from build123d import *

# Parameters (mm, degrees)
SKETCH1_W             = 74.422
SKETCH1_H             = 50.8
BOSS_EXTRUDE1_DEPTH   = 6.35
SKETCH2_R             = 3.175
CUT_EXTRUDE1_DEPTH    = 64.289975675
SKETCH3_R             = 4.7625
CUT_EXTRUDE2_DEPTH    = 64.289975675
F_8_CLEARANCE_HOLE1_D = 4.4958
SKETCH6_R             = 3.429
CUT_EXTRUDE3_DEPTH    = 4.572
SKETCH7_R             = 1.5875
CUT_EXTRUDE4_DEPTH    = 46.498802413
BODY_MOVE_COPY3_ANGLE = 180


with BuildPart() as part:
    # Sketch1 → Boss-Extrude1 (new body)
    with BuildSketch(Plane(origin=(0, 0, 0), x_dir=(1, 0, 0), z_dir=(0, 1, 0))):
        Rectangle(SKETCH1_W, SKETCH1_H)
    extrude(amount=BOSS_EXTRUDE1_DEPTH)

    # Sketch2 → Cut-Extrude1 (cut, through all)
    with BuildSketch(Plane.XY.offset(25.4)):
        with Locations((-24.511, 0)):
            Circle(SKETCH2_R)
        with Locations((26.289, 0)):
            Circle(SKETCH2_R)
    extrude(amount=-CUT_EXTRUDE1_DEPTH, mode=Mode.SUBTRACT)

    # Sketch3 → Cut-Extrude2 (cut, through all)
    with BuildSketch(Plane.XY.offset(25.4)):
        with Locations((-9.525, 0)):
            Circle(SKETCH3_R)
        with Locations((9.525, 0)):
            Circle(SKETCH3_R)
    extrude(amount=-CUT_EXTRUDE2_DEPTH, mode=Mode.SUBTRACT)

    # #8 Clearance Hole1 (through all)
    with Locations(Plane(origin=(0, 6.35, 0), x_dir=(1, 0, 0), z_dir=(0, 1, 0))):
        with Locations((-32.4485, 12.7), (-32.4485, -12.7), (-17.399, -12.7), (0, -12.7), (17.399, -12.7), (32.4485, -12.7), (32.4485, 12.7), (17.399, 12.7), (0, 12.7), (-17.399, 12.7)):
            Hole(F_8_CLEARANCE_HOLE1_D / 2)

    # Sketch6 → Cut-Extrude3 (cut)
    with BuildSketch(Plane(origin=(0, 6.35, 0), x_dir=(1, 0, 0), z_dir=(0, 1, 0))):
        with Locations(Location((-32.4485, 12.7, 0), (0, 0, 270))):
            Circle(SKETCH6_R)
        with Locations(Location((-17.399, 12.7, 0), (0, 0, 270))):
            Circle(SKETCH6_R)
        with Locations(Location((0, 12.7, 0), (0, 0, 270))):
            Circle(SKETCH6_R)
        with Locations(Location((17.399, 12.7, 0), (0, 0, 270))):
            Circle(SKETCH6_R)
        with Locations(Location((32.4485, 12.7, 0), (0, 0, 270))):
            Circle(SKETCH6_R)
        with Locations(Location((32.4485, -12.7, 0), (0, 0, 270))):
            Circle(SKETCH6_R)
        with Locations(Location((17.399, -12.7, 0), (0, 0, 270))):
            Circle(SKETCH6_R)
        with Locations(Location((0, -12.7, 0), (0, 0, 270))):
            Circle(SKETCH6_R)
        with Locations(Location((-17.399, -12.7, 0), (0, 0, 270))):
            Circle(SKETCH6_R)
        with Locations(Location((-32.4485, -12.7, 0), (0, 0, 270))):
            Circle(SKETCH6_R)
    extrude(amount=-CUT_EXTRUDE3_DEPTH, mode=Mode.SUBTRACT)

    # Sketch7 → Cut-Extrude4 (cut, through all)
    with BuildSketch(Plane(origin=(0, 6.35, 0), x_dir=(1, 0, 0), z_dir=(0, 1, 0))):
        with Locations(Location((0, 0, 0), (0, 0, 270))):
            Circle(SKETCH7_R)
    extrude(amount=-CUT_EXTRUDE4_DEPTH, mode=Mode.SUBTRACT)


with BuildPart() as part_1:
    # Body-Move/Copy3: moved
    add(part.part.moved(Location((0, 0, 0))).rotate(Axis((0, 3.175, 0), (0.7071067811865488, 0, -0.7071067811865462)), BODY_MOVE_COPY3_ANGLE))


solid = part_1.part
Geometry check sheet. Reference: the model listing, model coordinates, mm. A direction names the side the tool comes from. Give positions to 0.01 mm unless a question says otherwise; leave off trailing zeros. Order: outer loops, then holes, each group sorted by start corner. A loop starts at its lowest first (then second) coordinate and runs counter-clockwise, first axis right, second up.
1) Material ranges on probe 1 along X at (y, z) = (1.5, -17.5); probe 2 along X at (y, z) = (3.75, -0.5); probe 3 along Z at (x, y) = (-21, 4.75), recorded low to high.
Results are:
probe 1: x = -25.4 to -16.13, -9.27 to 9.27, 16.13 to 25.4
probe 2: x = -25.4 to -16.09, -9.31 to -1.51, 1.51 to 9.31, 16.09 to 25.4
probe 3: z = -37.21 to -29.03, -23.55 to -14.01, -5.04 to 5.04, 14.01 to 21.77, 27.25 to 37.21
2) Cross-section at A-A (z = 0). Record the boundary of the cut face in (x, y).
Results are:
outline: (-25.4, 0) - (-16.13, 0) - (-16.13, 4.57) - (-14.95, 4.57) - (-14.95, 6.35) - (-25.4, 6.35) - close; (-10.45, 4.57) - (-9.27, 4.57) - (-9.27, 0) - (-1.59, 0) - (-1.59, 6.35) - (-10.45, 6.35) - close; (1.59, 0) - (9.27, 0) - (9.27, 4.57) - (10.45, 4.57) - (10.45, 6.35) - (1.59, 6.35) - close; (14.95, 4.57) - (16.13, 4.57) - (16.13, 0) - (25.4, 0) - (25.4, 6.35) - (14.95, 6.35) - close
3) Gauge pin test, flat ends, axial feed: pin 1 (5 mm diameter, centred on x = 12.7, z = -32.45, fed in from +Y); pin 2 (3.5 mm diameter, centred on x = -12.5, z = -1, fed in from -Y). Record the tip position at first contact, or that the pin passes through.
Results are:
pin 1: stops at y = 6.35
pin 2: stops at y = 4.57
4) Cross-section at B-B (z = 16.5). Record the boundary of the cut face in (x, y), then the cut area to 3 significant figures.
Results are:
outline: (-25.4, 0) - (-16.01, 0) - (-16.01, 4.57) - (-14.76, 4.57) - (-14.76, 6.35) - (-25.4, 6.35) - close; (-10.64, 4.57) - (-9.39, 4.57) - (-9.39, 0) - (9.39, 0) - (9.39, 4.57) - (10.64, 4.57) - (10.64, 6.35) - (-10.64, 6.35) - close; (14.76, 4.57) - (16.01, 4.57) - (16.01, 0) - (25.4, 0) - (25.4, 6.35) - (14.76, 6.35) - close
area: 247 mm2
5) Tool access check on faces 3 (the cylindrical face through (12.799, 5.473, 15.153)), 4 (the flat face through (-13, 4.572, 20)). Record the directions out of +Z, -Z, +X, -X, +Y, -Y that give a thin tool (end or side, any length) a straight path to the whole face; none if there is none.
Results are:
face 3: +Y, -Y
face 4: -Y
6) Cross-section at C-C (x = -12.7). Give the number of separate pieces and of enclosed holes in the cut face, then the cut area to 3 significant figures.
Results are:
separate pieces: 6
enclosed holes: 0
area: 173 mm2
7) Draft check along X on faces 1 (the cylindrical face through (-0.356, 3.176, 24.441)), 2 (the cylindrical face through (-12.254, 2.254, -35.848)). Enter one of: released by +X, released by -X, zero draft, split by the parting line, or undercut.
Results are:
face 1: zero draft
face 2: undercut
